Autodesk Inventor part; units mm, degrees
ref_plane "YZ Plane" through (0, 0, 0) normal (1, 0, 0) x (0, 1, 0)
ref_plane "XZ Plane" through (0, 0, 0) normal (0, 1, 0) x (-1, 0, 0)
ref_plane "XY Plane" through (0, 0, 0) normal (0, 0, 1) x (1, 0, 0)
sketch "Sketch1" plane through (0, 0, 0) normal (0, 0, 1) x (1, 0, 0)
  line L0 (0, 0) -> (69, 0)
  line L1 (69, 0) -> (69, 64)
  line L2 (69, 64) -> (0, 64)
  line L3 (0, 64) -> (0, 0)
  dimension "d0" = 69
  dimension "d1" = 64
extrude "Extrusion1" add sketch "Sketch1" along normal blind 37
sketch "Sketch2" plane through (0, 0, 37) normal (0, 0, 1) x (1, 0, 0)
  line L0 (69, 64) -> (0, 64)
  line L1 (69, 0) -> (69, 64)
  line L2 (0, 64) -> (69, 64)
  line L3 (69, 64) -> (69, 0)
  line L4 (69, 0) -> (0, 0)
  line L5 (0, 0) -> (0, 64)
  line L6 (3, 3) -> (66, 3)
  line L7 (66, 3) -> (66, 61)
  line L8 (66, 61) -> (3, 61)
  line L9 (3, 61) -> (3, 3)
  dimension "d4" = 3
extrude "Extrusion2" cut sketch "Sketch2" against normal blind 34 contours L9 L8 L7 L6
sketch "Sketch3" plane through (0, 0, 0) normal (0, -1, 0) x (1, 0, 0)
  line L0 (3, 37) -> (3, 3)
  line L1 (66, 37) -> (66, 3)
  line L2 (3, 37) -> (66, 37)
  line L3 (66, 37) -> (66, 34)
  line L4 (66, 34) -> (3, 34)
  line L5 (3, 34) -> (3, 37)
  point P0 (0, 0)
  point P1 (3, 34)
  dimension "d7" = 3
extrude "Extrusion3" cut sketch "Sketch3" against normal up to surface (3 mm away)
sketch "Sketch4" plane through (0, 0, 0) normal (0, -1, 0) x (1, 0, 0)
  line L0 (3, 34) -> (66, 34)
  line L1 (34.5, 34) -> (67.5, 34)
  line L2 (67.5, 34) -> (1.5, 34)
  line L3 (1.5, 34) -> (1.5, 35.44)
  line L4 (1.5, 35.44) -> (67.5, 35.44)
  line L5 (67.5, 35.44) -> (67.5, 34)
  point P0 (0, 0)
  dimension "d10" = 33
  dimension "d11" = 66
  dimension "d12" = 1.44
extrude "Extrusion4" cut sketch "Sketch4" against normal blind 62.9
properties part number "TOP"
Here's how the part is built. I have some questions about the finished solid (model axes, mm). A direction names the side the tool comes from. Give positions to 0.01 mm unless a question says otherwise; leave off trailing zeros. Loops run counter-clockwise (first coordinate to the right, second up) from the corner with the lowest first, then second, coordinate; pieces in that order, holes last. Notation, with made-up numbers: (13, 81.5) -> (32, 81.5) arc R34 cw to (32, 120.5) -> close; hole circle Ø8 at (47, -31). An arc over 180 degrees is marked (long way). One line per item, written item: value.
Q1. Suppose I cut it at A-A on z = 26. Please give me the cut outline in (x, y).
Answers follow:
outline: (0, 0) -> (69, 0) -> (69, 64) -> (0, 64) -> close; hole (3, 3) -> (66, 3) -> (66, 61) -> (3, 61) -> close
Q2. Suppose I cut it at C-C on y = 16. Please give me the cut outline in (x, z), then the cut area to 3 significant figures.
Answers follow:
outline: (0, 0) -> (69, 0) -> (69, 37) -> (66, 37) -> (66, 35.44) -> (67.5, 35.44) -> (67.5, 34) -> (66, 34) -> (66, 3) -> (3, 3) -> (3, 34) -> (1.5, 34) -> (1.5, 35.44) -> (3, 35.44) -> (3, 37) -> (0, 37) -> close
area: 407 mm^2
Q3. Suppose I cut it at B-B on x = 52. Please give me the cut outline in (y, z), then the cut area to 3 significant figures.
Answers follow:
outline: (0, 0) -> (64, 0) -> (64, 37) -> (61, 37) -> (61, 35.44) -> (62.9, 35.44) -> (62.9, 34) -> (61, 34) -> (61, 3) -> (3, 3) -> (3, 34) -> (0, 34) -> close
area: 384 mm^2
Q4. I'm going to push flat-ended pins straight in: pin 1 Ø4 at (x, y) = (29.5, 28.5) entering from +Z; pin 2 Ø1.2 at (x, z) = (45, 36) entering from -Y; pin 3 Ø0.7 at (x, z) = (30.5, 34.5) entering from -Y. Where does each tip first touch, or does it pass through?
Answers follow:
pin 1: z = 3
pin 2: y = 61
pin 3: y = 62.9
Q5. We'd pull the mould along Z, two halves only. Please class faces 4 (the face through (34, 32, 0)), 5 (the face through (32, 62, 34)), 6 (the face through (35, 61, 36)): pulls with the +Z half, pulls with the -Z half, needs draft (parallel to the pull), parting line crosses it, or undercut.
Answers follow:
face 4: pulls with the -Z half
face 5: undercut
face 6: needs draft
Q6. If I drill on line 1 along X through (y, z) = (58.5, 32); line 2 along Y through (x, z) = (8, 25); line 3 along Z through (x, y) = (55, 11), over which ranges is the centre line in solid material (lowest first)?
Answers follow:
line 1: 0 to 3, 66 to 69
line 2: 0 to 3, 61 to 64
line 3: 0 to 3
Q7. On a 3-axis mill with a long thin cutter (end or side, diameter ignored), from which of +Z, -Z, +X, -X, +Y, -Y can I reach the whole of each face in a straight line? I mean faces 1 (the face through (66, 30, 36)), 2 (the face through (34, 62, 35.44)), 3 (the face through (35, 61, 19)). Say none if no direction works.
Answers follow:
face 1: +Z, -Y
face 2: -Y
face 3: +Z
